The model under review builds one solid part; all positions refer to its coordinate system, in mm. A direction names the side the tool comes from. Give positions to 0.01 mm unless a question says otherwise; leave off trailing zeros. Loops run counter-clockwise (first coordinate to the right, second up) from the corner with the lowest first, then second, coordinate; pieces in that order, holes last. Notation, with made-up numbers: M 50,0 L 62,0 A18 cw 62,9 Z; hole C 0.5,-40 d2. An arc over 180 degrees is marked long. Write item = value, one per line. Start each with the question number.
1. For faces 1 (the face through (9.755, -0.295, -10.693)), 2 (the face through (24.75, 3, -14)), 3 (the face through (24, -2, -14)), 4 (the face through (-24.75, -3, -14)), 5 (the face through (-24, 2, -14)), list the 3-axis set-ups (+Z, -Z, +X, -X, +Y, -Y) from which the entire face can be reached by the end or side of a thin tool; tool diameter is ignored.
2. We need section C-C on y = -1.5. Give the boundary of the cut face in (x, z).
3. Wall thickness on line 1 along X through (y, z) = (-1.5, -5.5); line 2 along Y through (x, z) = (-22.5, -5); line 3 along X through (y, z) = (-1, -5.5): over which ranges is each line inside the solid? List them lowest first. Write a range as from..to.
4. For pin 1 (0.8 mm diameter, centred on x = 24, z = -12.5, fed in from +Y), flat-tipped, find the tip position at first contact; note if it passes through.
5. We need section D-D on x = 8.5. Give the boundary of the cut face in (y, z).
6. Draft analysis for pull direction X (two halves, no side actions). For faces 6 (the face through (21.25, 0.04, -13.8)), 7 (the face through (-21.25, -0.04, -13.8)), 8 (the face through (24, 2, -14)), 9 (the face through (-9.755, 0.295, -10.693)), state which applies: pulls with the +X half, pulls with the -X half, needs draft (parallel to the pull), parting line crosses it, or undercut.
7. We need section B-B on z = -9.75. Give the boundary of the cut face in (x, y).
8. We need section A-A on z = -25.75. Give the boundary of the cut face in (x, y), then the cut area to 3 significant figures.
from build123d import *

# Parameters (mm, degrees)
EXTRUDE_1_DEPTH   = 28
EXTRUDE_1_2_DEPTH = 28
EXTRUDE_START     = -17.75
EXTRUDE_2_DEPTH   = 35.5


with BuildPart() as part:
    # Sketch 1 → Extrude 1 (new body)
    with BuildSketch(Plane.XY):
        with BuildLine():
            Line((-23.25, 2), (-24.75, 2))
            Line((-24.75, 2), (-24.75, 3.872983346))
            ThreePointArc((-24.75, 3.872983346), (-9.75, 0), (-24.75, -3.872983346))
            Line((-24.75, -3.872983346), (-24.75, -2))
            Line((-24.75, -2), (-23.25, -2))
            ThreePointArc((-23.25, -2), (-21.25, 0), (-23.25, 2))
        make_face()
    extrude(amount=-EXTRUDE_1_DEPTH)



with BuildPart() as body_2:
    # Sketch 1 → Extrude 1 2 (new body)
    with BuildSketch(Plane.XY):
        with BuildLine():
            Line((23.25, -2), (24.75, -2))
            Line((24.75, -2), (24.75, -3.872983346))
            ThreePointArc((24.75, -3.872983346), (9.75, 0), (24.75, 3.872983346))
            Line((24.75, 3.872983346), (24.75, 2))
            Line((24.75, 2), (23.25, 2))
            ThreePointArc((23.25, 2), (21.25, 0), (23.25, -2))
        make_face()
    extrude(amount=-EXTRUDE_1_2_DEPTH)


with BuildPart() as part_1:
    add(part.part)

    add(body_2.part)  # Extrude 2 merges body 2
    # Sketch 2 → Extrude 2 (add)
    with BuildSketch(Plane(origin=(0, 0, 0), x_dir=(0, 0, -1), z_dir=(1, 0, 0)).offset(EXTRUDE_START)):
        with BuildLine():
            Line((28, -8), (28, 8))
            Line((28, 8), (22, 8))
            ThreePointArc((22, 8), (14, 0), (22, -8))
            Line((22, -8), (28, -8))
        make_face()
    extrude(amount=EXTRUDE_2_DEPTH)


solid = part_1.part
Final values:
q1.face_1 = +Z
q1.face_2 = +Z, -Z, +X, +Y, -Y
q1.face_3 = +Z, -Z, +X
q1.face_4 = +Z, -Z, -X, +Y, -Y
q1.face_5 = +Z, -Z, -X
q2.outline = M -21.93,-28 L 21.93,-28 L 21.93,0 L 9.89,0 L 9.89,-14.14 L -9.89,-14.14 L -9.89,0 L -21.93,0 Z
q3.line_1 = -21.93..-9.89, 9.89..21.93
q3.line_2 = -6.44..-1.85, 1.85..6.44
q3.line_3 = -21.52..-9.81, 9.81..21.52
q4.pin_1 = 5.46
q5.outline = M -8,-28 L 8,-28 L 8,-22 A8 ccw -8,-22 Z
q6.face_6 = pulls with the +X half
q6.face_7 = pulls with the -X half
q6.face_8 = needs draft
q6.face_9 = undercut
q7.outline = M -24.75,-3.87 A8 ccw long -24.75,3.87 L -24.75,2 L -23.25,2 A2 cw -23.25,-2 L -24.75,-2 Z; M 23.25,-2 A2 cw 23.25,2 L 24.75,2 L 24.75,3.87 A8 ccw long 24.75,-3.87 L 24.75,-2 Z
q8.outline = M -24.75,-3.87 A8 ccw -17.75,-8 L 17.75,-8 A8 ccw 24.75,-3.87 L 24.75,-2 L 23.25,-2 A2 cw 23.25,2 L 24.75,2 L 24.75,3.87 A8 ccw 17.75,8 L -17.75,8 A8 ccw -24.75,3.87 L -24.75,2 L -23.25,2 A2 cw -23.25,-2 L -24.75,-2 Z
q8.area = 734 mm²
